Check sheet for the modelled part. Datum: model origin and axes. Units: mm. A direction names the side the tool comes from. Give positions to 0.01 mm unless a question says otherwise; leave off trailing zeros. Order: outer loops, then holes, each group sorted by start corner. A loop starts at its lowest first (then second) coordinate and runs counter-clockwise, first axis right, second up. Notation, with made-up numbers: (-9.5, -5.5) -> (14.5, -5.5) arc R19 ccw to (14.5, 16.5) -> close; hole circle Ø11 at (59.5, 57.25). An arc over 180 degrees is marked (long way). Answer in a Markdown table with one row per item. Add a question column.
(1) Cross-section at C-C (z = 8.5). Record the cut outline in (x, y).
(2) Cross-section at D-D (x = 4). Record the cut outline in (y, z), then the cut area to 4 significant figures.
(3) Set-up check for faces 4 (the face through (0, 32.527, 11)), 5 (the face through (-4.887, 33, 20)), 6 (the face through (7, -24.043, 5)), 7 (the face through (7.813, 33, 20)), 8 (the face through (0, 34.527, 10)): record each of +Z, -Z, +X, -X, +Y, -Y from which the full face is reachable in a straight line by a thin tool's end or side.
(4) Thickness scan on L1, parallel to X at y = 32, z = 21; L2, parallel to X at y = -18.5, z = 4.75; L3, parallel to Y at x = -1, z = 4.25. Record the ranges inside material, lowest first. Write a range as [from, to].
(5) Release check for a two-part mould opening along X. For faces 1 (the face through (11, 32.527, 23)), 2 (the face through (0, 27.457, 2)), 3 (the face through (15.613, 4, 5)) record: released by +X, released by -X, zero draft, split by the parting line, or undercut.
(6) Go/stop test with flat-tipped pins: pin 1 (3 mm diameter, centred on x = 10.5, z = 22.5, fed in from -Y); pin 2 (7.5 mm diameter, centred on x = -4, z = 12.5, fed in from -Y); pin 3 (1 mm diameter, centred on x = 2.5, y = 34, fed in from +Z); pin 4 (1.5 mm diameter, centred on y = 32.5, z = 18, fed in from -X). Record where each tip stops, or that it passes through.
(7) Cross-section at A-A (z = 19.25). Record the cut outline in (x, y).
(8) Cross-section at B-B (y = -17.5). Record the cut outline in (x, z).
```python
from build123d import *

# Parameters (mm, degrees)
F0_W     = 30.5
F0_H     = 60.57
F0_W_2   = 1.524
F0_H_2   = 4
F1_DEPTH = 10
F0_W_3   = 26.5
F0_H_3   = 5.07
F2_DEPTH = 5
F3_W     = 26.5
F3_H     = 2
F4_DEPTH = 15
F5_W     = 1
F5_H     = 1.5
F6_DEPTH = 25.4
F7_R     = 0.5
F8_W     = 8
F8_H     = 7.14287
F9_DEPTH = 10


with BuildPart() as f1:
    # F0 (on Top) → F1 (new body)
    with BuildSketch(Plane.XY):
        with Locations((0.363031, 4.242457)):
            Rectangle(F0_W, F0_H)
        Polygon((-12.886969, 27.457457), (-12.886969, 32.527457), (13.613031, 32.527457), (13.613031, 27.457457), (13.613031, -24.042543), (0.637031, -24.042543), (-0.886969, -24.042543), (-12.886969, -24.042543), align=None, mode=Mode.SUBTRACT)
        with Locations((-0.124969, -22.042543)):
            Rectangle(F0_W_2, F0_H_2)
    extrude(amount=F1_DEPTH)

    # F0 (on Top) → F2 (join)
    with BuildSketch(Plane.XY):
        with Locations((0.363031, 29.992457)):
            Rectangle(F0_W_3, F0_H_3)
    extrude(amount=F2_DEPTH)

    # F3 (on face) → F4 (join)
    with BuildSketch(Plane.XY.offset(10)):
        with Locations((0.363031, 33.527457)):
            Rectangle(F3_W, F3_H)
    extrude(amount=F4_DEPTH)

    # F5 (on face) → F6 (join)
    with BuildSketch(Plane.YZ.offset(13.613031)):
        with Locations((32.027457, 20.75)):
            Rectangle(F5_W, F5_H)
    extrude(amount=-F6_DEPTH)

    # F7
    f7_edges = [f1.edges().sort_by_distance(p)[0] for p in [
        (0.913031, 31.527457, 21.5),
        (0.913031, 31.527457, 20),
    ]]
    fillet(f7_edges, radius=F7_R)

    # F8 (on face) → F9 (cut)
    with BuildSketch(Plane.XY.offset(25)):
        with Locations((-8.886969, 30.956022)):
            Rectangle(F8_W, F8_H)
        with Locations((3.813031, 30.956022)):
            Rectangle(F8_W, F8_H)
    extrude(amount=-F9_DEPTH, mode=Mode.SUBTRACT)


solid = f1.part
```
Answer below:
| question | item | result |
|---|---|---|
| 1 | outline | (-14.89, -26.04) -> (15.61, -26.04) -> (15.61, 34.53) -> (-14.89, 34.53) -> close; hole (-12.89, -24.04) -> (-0.89, -24.04) -> (-0.89, -20.04) -> (0.64, -20.04) -> (0.64, -24.04) -> (13.61, -24.04) -> (13.61, 32.53) -> (-12.89, 32.53) -> close |
| 2 | outline | (-26.04, 0) -> (-24.04, 0) -> (-24.04, 10) -> (-26.04, 10) -> close; (27.46, 0) -> (34.53, 0) -> (34.53, 15) -> (32.53, 15) -> (32.53, 5) -> (27.46, 5) -> close |
| 2 | area | 75.35 mm² |
| 3 | face 4 | none |
| 3 | face 5 | +Z, -X, +Y, -Y |
| 3 | face 6 | +Z, -Z |
| 3 | face 7 | +Z, +Y, -Y |
| 3 | face 8 | +Z, -Z, +X, -X, +Y |
| 4 | L1 | x = [-4.89, -0.19], [7.81, 13.61] |
| 4 | L2 | x = [-14.89, -12.89], [13.61, 15.61] |
| 4 | L3 | y = [-26.04, -24.04], [27.46, 34.53] |
| 5 | face 1 | zero draft |
| 5 | face 2 | undercut |
| 5 | face 3 | released by +X |
| 6 | pin 1 | stops at y = 31.53 |
| 6 | pin 2 | stops at y = -26.04 |
| 6 | pin 3 | stops at z = 15 |
| 6 | pin 4 | stops at x = -4.89 |
| 7 | outline | (-4.89, 32.53) -> (-0.19, 32.53) -> (-0.19, 34.53) -> (-4.89, 34.53) -> close; (7.81, 32.53) -> (13.61, 32.53) -> (13.61, 34.53) -> (7.81, 34.53) -> close |
| 8 | outline | (-14.89, 0) -> (-12.89, 0) -> (-12.89, 10) -> (-14.89, 10) -> close; (13.61, 0) -> (15.61, 0) -> (15.61, 10) -> (13.61, 10) -> close |
